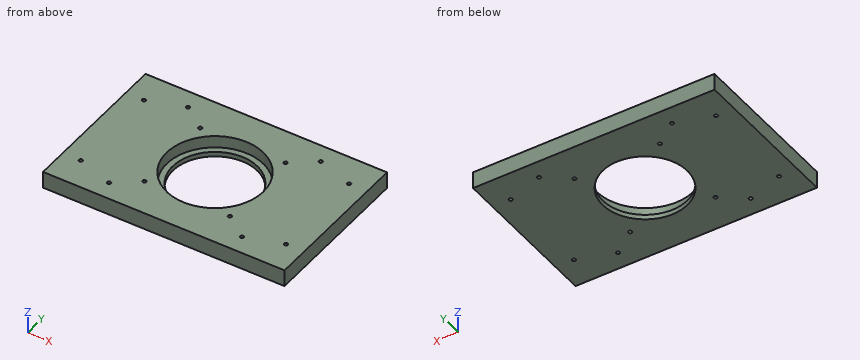
from build123d import *

# Parameters (mm, degrees)
SKETCH_W     = 200
SKETCH_H     = 130
SKETCH_R     = 35
SKETCH_R_2   = 1.5
PAD_DEPTH    = 14
SKETCH001_R  = 40
POCKET_DEPTH = 10


with BuildPart() as part:
    # Sketch → Pad (new body)
    with BuildSketch(Plane.XY):
        with Locations((100, 65)):
            Rectangle(SKETCH_W, SKETCH_H)
        with Locations((100, 65)):
            Circle(SKETCH_R, mode=Mode.SUBTRACT)
        with Locations((45, 115)):
            Circle(SKETCH_R_2, mode=Mode.SUBTRACT)
        with Locations((45, 15)):
            Circle(SKETCH_R_2, mode=Mode.SUBTRACT)
        with Locations((155, 115)):
            Circle(SKETCH_R_2, mode=Mode.SUBTRACT)
        with Locations((155, 15)):
            Circle(SKETCH_R_2, mode=Mode.SUBTRACT)
        with Locations((15, 105)):
            Circle(SKETCH_R_2, mode=Mode.SUBTRACT)
        with Locations((15, 25)):
            Circle(SKETCH_R_2, mode=Mode.SUBTRACT)
        with Locations((185, 105)):
            Circle(SKETCH_R_2, mode=Mode.SUBTRACT)
        with Locations((185, 25)):
            Circle(SKETCH_R_2, mode=Mode.SUBTRACT)
        with Locations((135.355339, 100.355339)):
            Circle(SKETCH_R_2, mode=Mode.SUBTRACT)
        with Locations((64.644661, 29.644661)):
            Circle(SKETCH_R_2, mode=Mode.SUBTRACT)
        with Locations((64.64463, 100.35537)):
            Circle(SKETCH_R_2, mode=Mode.SUBTRACT)
        with Locations((135.355307, 29.644693)):
            Circle(SKETCH_R_2, mode=Mode.SUBTRACT)
    extrude(amount=PAD_DEPTH)

    # Sketch001 (on Face19 of Pad) → Pocket (cut)
    with BuildSketch(Plane.XY.offset(14)):
        with Locations((100, 65)):
            Circle(SKETCH001_R)
    extrude(amount=-POCKET_DEPTH, mode=Mode.SUBTRACT)


solid = part.part
Part model, mm, in its own coordinate system. Give positions to 0.01 mm unless a question says otherwise; leave off trailing zeros. Order: outer loops, then holes, each group sorted by start corner. A loop starts at its lowest first (then second) coordinate and runs counter-clockwise, first axis right, second up. Notation, with made-up numbers: (29, 21) -> (62, 21) arc R27 cw to (62, 56) -> close; hole circle Ø3 at (24, 9). An arc over 180 degrees is marked (long way). Use one line per item in the form item = value.
(1) Drill centre lines: line 1 (X direction, y = 115, z = 7.5); line 2 (Y direction, x = 100, z = 2.9); line 3 (Y direction, x = 100, z = 4.5). Where is each one in solid material? Low to high. Write a range as from..to.
Solution:
line_1 = 0..43.5, 46.5..153.5, 156.5..200
line_2 = 0..30, 100..130
line_3 = 0..25, 105..130
(2) Saw through at B-B (x = 115.5). Write the cut outline in (y, z).
Solution:
outline = (0, 0) -> (33.62, 0) -> (33.62, 4) -> (28.13, 4) -> (28.13, 14) -> (0, 14) -> close; (96.38, 0) -> (130, 0) -> (130, 14) -> (101.87, 14) -> (101.87, 4) -> (96.38, 4) -> close
(3) Saw through at C-C (z = 8.5). Count the separate pieces of the cut face and the enclosed holes in it, then the cut area to 3 significant figures.
Solution:
separate_pieces = 1
enclosed_holes = 13
area = 20,900 mm²
(4) Flat gauge pin, fed straight in: P1, Ø2.5, axis at x = 155, y = 15, coming from the -Z side. Where does the tip first touch, or does it go through?
Solution:
P1 = through
(5) Saw through at A-A (y = 65). Write the cut outline in (x, z), then the cut area to 3 significant figures.
Solution:
outline = (0, 0) -> (65, 0) -> (65, 4) -> (60, 4) -> (60, 14) -> (0, 14) -> close; (135, 0) -> (200, 0) -> (200, 14) -> (140, 14) -> (140, 4) -> (135, 4) -> close
area = 1,720 mm²
